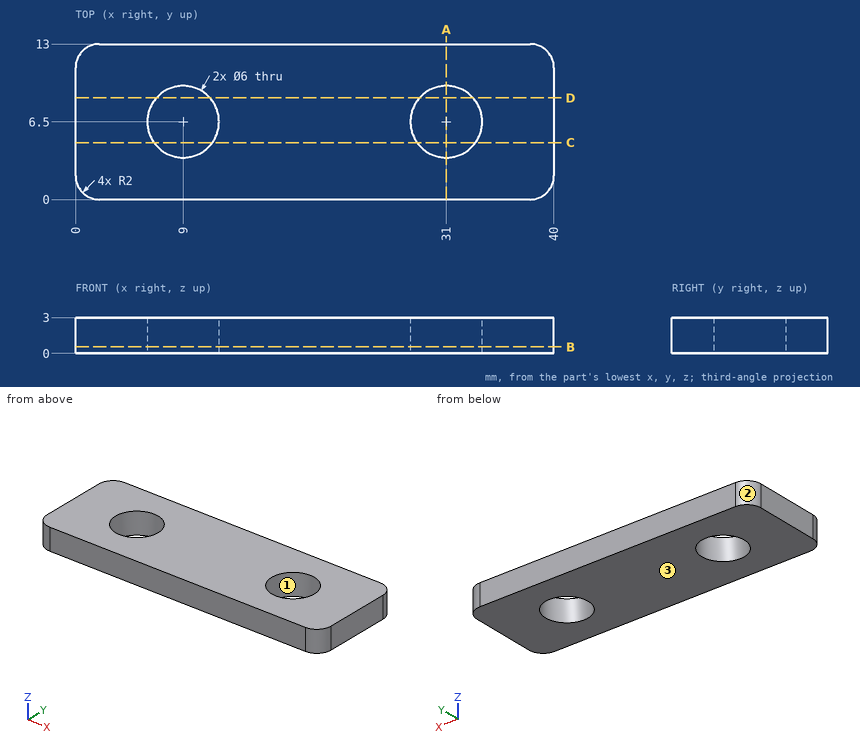
Drawing for the job (mm, zero at the part's lowest x, y, z). Give positions to 0.01 mm unless a question says otherwise; leave off trailing zeros. Order: outer loops, then holes, each group sorted by start corner. A loop starts at its lowest first (then second) coordinate and runs counter-clockwise, first axis right, second up. Notation, with made-up numbers: M 2,64.25 L 23,64.25 A23 cw 23,103.25 Z; hole C 44.25,63 d4. An arc over 180 degrees is marked long. Use a Markdown table: item, result. Add a question column.
(1) Saw through at B-B, the plane z = 0.55. Give the cut face in (x, y).
(2) Saw through at A-A, the plane x = 31. Give the cut face in (y, z), and give its area (3 significant figures).
(3) Saw through at C-C, the plane y = 4.75. Give the cut face in (x, z).
(4) Probe line 1 along Y through (x, z) = (9, 1.95); line 2 along X through (y, z) = (4.75, 1.5); line 3 along X through (y, z) = (4.5, 0.6). List the from-to ranges inside material, lowest first. Write a range as [from, to].
(5) Drop a flat-ended pin along its axis: P1, Ø2, axis at x = 8, y = 10.5, coming from the -Z side. Give the stop position or say it passes through.
(6) Saw through at D-D, the plane y = 8.5. Give the cut face in (x, z).
(7) Mould opens along Y. For the marked faces 1, 2 and 3 say: +Y half, -Y half, draft (parallel to the pull), parting line (faces both ways), or undercut.
Answer key:
| question | item | result |
|---|---|---|
| 1 | outline | M 0,2 A2 ccw 2,0 L 38,0 A2 ccw 40,2 L 40,11 A2 ccw 38,13 L 2,13 A2 ccw 0,11 Z; hole C 9,6.5 d6; hole C 31,6.5 d6 |
| 2 | outline | M 0,0 L 3.5,0 L 3.5,3 L 0,3 Z; M 9.5,0 L 13,0 L 13,3 L 9.5,3 Z |
| 2 | area | 21.0 mm^2 |
| 3 | outline | M 0,0 L 6.56,0 L 6.56,3 L 0,3 Z; M 11.44,0 L 28.56,0 L 28.56,3 L 11.44,3 Z; M 33.44,0 L 40,0 L 40,3 L 33.44,3 Z |
| 4 | line 1 | [0, 3.5], [9.5, 13] |
| 4 | line 2 | [0, 6.56], [11.44, 28.56], [33.44, 40] |
| 4 | line 3 | [0, 6.76], [11.24, 28.76], [33.24, 40] |
| 5 | P1 | z = 0 |
| 6 | outline | M 0,0 L 6.76,0 L 6.76,3 L 0,3 Z; M 11.24,0 L 28.76,0 L 28.76,3 L 11.24,3 Z; M 33.24,0 L 40,0 L 40,3 L 33.24,3 Z |
| 7 | face 1 | undercut |
| 7 | face 2 | +Y half |
| 7 | face 3 | draft |
